Verification items for the finished model (mm, model axes). A direction names the side the tool comes from. Give positions to 0.01 mm unless a question says otherwise; leave off trailing zeros. Order: outer loops, then holes, each group sorted by start corner. A loop starts at its lowest first (then second) coordinate and runs counter-clockwise, first axis right, second up. Notation, with made-up numbers: (-23, 68.25) - (35, 68.25) arc R31 cw to (35, 92.25) - close; hole circle Ø3 at (-18, -14.5). An arc over 180 degrees is marked (long way). Answer as a JSON object with one key per item and string values. Group by question number.
(1) Section check A-A (z = 186). Record the boundary of the cut face in (x, y).
(2) Thickness scan on line 1 (X direction, y = 0.5, z = 274.5); line 2 (Y direction, x = -3.5, z = 31.5); line 3 (X direction, y = -2.5, z = 189). Record the ranges inside material, lowest first.
(3) Depth check by flat-ended pin: pin 1 Ø1.5 at (x, z) = (-21.5, 146.5) entering from -Y; pin 2 Ø6 at (x, z) = (13, 75) entering from +Y; pin 3 Ø1.5 at (x, y) = (13.5, 21) entering from -Z. Enter the tip coordinate at first touch or a pass-through.
(4) Mould release check, pull along Y, two halves, no side actions. Record for faces 1 (the face through (4, -4, 292.1)), 2 (the face through (4.812, 0, 144)), 3 (the face through (-6.883, -30.995, 144.183)), 4 (the face through (-2.44, -4.148, 144.005)): +Y half, -Y half, draft (parallel to the pull), parting line (faces both ways), or undercut.
(5) Access from +Z, -Z, +X, -X, +Y, -Y to the whole of each face (thin tool, end or side, straight path). Record for faces 5 (the face through (4, -4, 0)), 6 (the face through (2.44, 4.148, 144.005)).
(6) Section check B-B (y = 0). Record the boundary of the cut face in (x, z), then the cut area to 3 significant figures.
```python
from build123d import *

# Parameters (mm, degrees)
SKETCH1_R           = 31.75
BOSS_EXTRUDE1_DEPTH = 292.1
FILLET1_R           = 12.7
FILLET2_R           = 12.7


with BuildPart() as part:
    # Sketch1 → Boss-Extrude1 (new body)
    with BuildSketch(Plane.XY):
        Circle(SKETCH1_R)
        Polygon((0, -5.55625), (4.81185365, -2.778125), (4.81185365, 2.778125), (0, 5.55625), (-4.81185365, 2.778125), (-4.81185365, -2.778125), align=None, mode=Mode.SUBTRACT)
    extrude(amount=BOSS_EXTRUDE1_DEPTH)

    # Fillet1
    fillet1_edges = [part.edges().sort_by_distance(p)[0] for p in [
        (-31.75, 0, 292.1),
    ]]
    fillet(fillet1_edges, radius=FILLET1_R)

    # Fillet2
    fillet2_edges = [part.edges().sort_by_distance(p)[0] for p in [
        (-31.75, 0, 0),
    ]]
    fillet(fillet2_edges, radius=FILLET2_R)


solid = part.part
```
Solutions:
{
 "1": {"outline": "circle Ø63.5 at (0, 0); hole (-4.81, -2.78) - (0, -5.56) - (4.81, -2.78) - (4.81, 2.78) - (0, 5.56) - (-4.81, 2.78) - close"},
 "2": {"line 1": "x = -31.75 to -4.81, 4.81 to 31.75", "line 2": "y = -31.56 to -3.54, 3.54 to 31.56", "line 3": "x = -31.65 to -4.81, 4.81 to 31.65"},
 "3": {"pin 1": "stops at y = -24.03", "pin 2": "stops at y = 30.13", "pin 3": "stops at z = 1.1"},
 "4": {"face 1": "draft", "face 2": "undercut", "face 3": "parting line", "face 4": "undercut"},
 "5": {"face 5": "-Z, +X, -X, +Y, -Y", "face 6": "+Z, -Z"},
 "6": {"outline": "(-31.75, 12.7) arc R12.7 ccw to (-19.05, 0) - (-4.81, 0) - (-4.81, 292.1) - (-19.05, 292.1) arc R12.7 ccw to (-31.75, 279.4) - close; (4.81, 0) - (19.05, 0) arc R12.7 ccw to (31.75, 12.7) - (31.75, 279.4) arc R12.7 ccw to (19.05, 292.1) - (4.81, 292.1) - close", "area": "15,600 mm2"}
}
